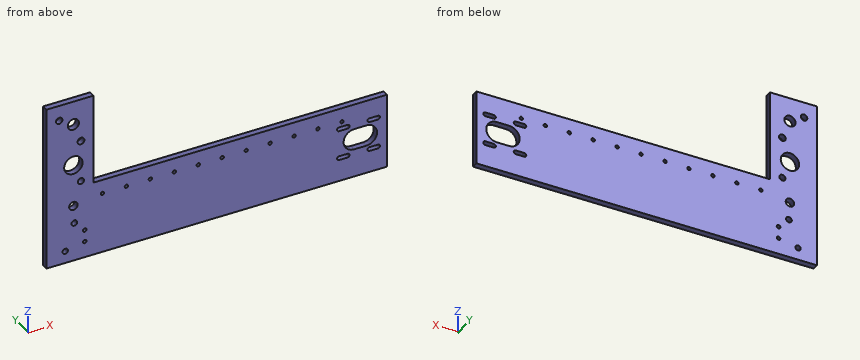
from build123d import *

# Parameters (mm, degrees)
BOSS_EXTRUDE1_DEPTH = 6.35
SKETCH2_R           = 2.979007601
CUT_EXTRUDE1_DEPTH  = 7.35
SKETCH3_R           = 4.400364859
SKETCH3_R_2         = 9.604356308
SKETCH3_R_3         = 5.866647912
SKETCH3_R_4         = 3.226485866
SKETCH3_R_5         = 3.595926688
SKETCH3_R_6         = 3.386947747
SKETCH3_R_7         = 2.817872048
SKETCH3_R_8         = 1.840203328
SKETCH3_R_9         = 1.930985623
CUT_EXTRUDE2_DEPTH  = 7.35
SKETCH4_R           = 1.778
CUT_EXTRUDE3_DEPTH  = 7.35


with BuildPart() as part:
    # Sketch1 → Boss-Extrude1 (new body)
    with BuildSketch(Plane(origin=(0, 0, 0), x_dir=(1, 0, 0), z_dir=(0, 1, 0))):
        Polygon((-177.8, -87.3125), (-177.8, 87.3125), (177.8, 87.3125), (177.8, 8.2677), (-128.5875, 8.2677), (-128.5875, -87.3125), align=None)
    extrude(amount=BOSS_EXTRUDE1_DEPTH)

    # Sketch2 → Cut-Extrude1 (cut, through all)
    with BuildSketch(Plane(origin=(0, 6.35, 0), x_dir=(1, 0, 0), z_dir=(0, 1, 0))):
        with BuildLine():
            Line((143.6116, 35.2552), (156.3116, 35.2552))
            ThreePointArc((156.3116, 35.2552), (167.4241, 46.3677), (156.3116, 57.4802))
            Line((156.3116, 57.4802), (143.6116, 57.4802))
            ThreePointArc((143.6116, 57.4802), (132.4991, 46.3677), (143.6116, 35.2552))
        make_face()
        with BuildLine():
            Line((159.4866, 60.1472), (168.376602437, 60.1472))
            ThreePointArc((168.376602437, 60.1472), (170.472102437, 62.2427), (168.376602437, 64.3382))
            Line((168.376602437, 64.3382), (159.486602437, 64.3382))
            ThreePointArc((159.486602437, 64.3382), (157.3911, 62.242701219), (159.4866, 60.1472))
        make_face()
        with BuildLine():
            ThreePointArc((159.486602437, 28.3972), (157.3911, 30.492698781), (159.4866, 32.5882))
            Line((159.4866, 32.5882), (168.376602437, 32.5882))
            ThreePointArc((168.376602437, 32.5882), (170.472102437, 30.4927), (168.376602437, 28.3972))
            Line((168.376602437, 28.3972), (159.486602437, 28.3972))
        make_face()
        with BuildLine():
            Line((127.7366, 60.1472), (136.626602437, 60.1472))
            ThreePointArc((136.626602437, 60.1472), (138.722102437, 62.2427), (136.626602437, 64.3382))
            Line((136.626602437, 64.3382), (127.736602437, 64.3382))
            ThreePointArc((127.736602437, 64.3382), (125.6411, 62.242701219), (127.7366, 60.1472))
        make_face()
        with BuildLine():
            Line((136.626602437, 28.3972), (127.736602437, 28.3972))
            ThreePointArc((127.736602437, 28.3972), (125.6411, 30.492698781), (127.7366, 32.5882))
            Line((127.7366, 32.5882), (136.626602437, 32.5882))
            ThreePointArc((136.626602437, 32.5882), (138.722102437, 30.4927), (136.626602437, 28.3972))
        make_face()
        with Locations((-148.4884, 46.3677)):
            Circle(SKETCH2_R)
    extrude(amount=-CUT_EXTRUDE1_DEPTH, mode=Mode.SUBTRACT)

    # Sketch3 → Cut-Extrude2 (cut, through all)
    with BuildSketch(Plane(origin=(0, 6.35, 0), x_dir=(1, 0, 0), z_dir=(0, 1, 0))):
        with Locations((-149.5425, 27.305)):
            Circle(SKETCH3_R)
        with Locations((-149.5425, -17.4625)):
            Circle(SKETCH3_R_2)
        with Locations((-149.5425, -62.23)):
            Circle(SKETCH3_R_3)
        with Locations((-141.63041575, 2.468910578)):
            Circle(SKETCH3_R_4)
        with Locations((-141.63041575, -41.536127476)):
            Circle(SKETCH3_R_5)
        with Locations((-164.313722824, -70.828896652)):
            Circle(SKETCH3_R_6)
        with Locations((-157.998667059, 74.512666328)):
            Circle(SKETCH3_R_7)
        with Locations((-137.701702146, 70.163316704)):
            Circle(SKETCH3_R_8)
        with Locations((-137.701702146, 57.549974441)):
            Circle(SKETCH3_R_9)
    extrude(amount=-CUT_EXTRUDE2_DEPTH, mode=Mode.SUBTRACT)

    # Sketch4 → Cut-Extrude3 (cut, through all)
    with BuildSketch(Plane(origin=(0, 6.35, 0), x_dir=(1, 0, 0), z_dir=(0, 1, 0))):
        with Locations((130.81, 23.1267)):
            Circle(SKETCH4_R)
        with Locations((105.81, 23.1267)):
            Circle(SKETCH4_R)
        with Locations((80.81, 23.1267)):
            Circle(SKETCH4_R)
        with Locations((55.81, 23.1267)):
            Circle(SKETCH4_R)
        with Locations((30.81, 23.1267)):
            Circle(SKETCH4_R)
        with Locations((5.81, 23.1267)):
            Circle(SKETCH4_R)
        with Locations((-19.19, 23.1267)):
            Circle(SKETCH4_R)
        with Locations((-44.19, 23.1267)):
            Circle(SKETCH4_R)
        with Locations((-69.19, 23.1267)):
            Circle(SKETCH4_R)
        with Locations((-94.19, 23.1267)):
            Circle(SKETCH4_R)
        with Locations((-119.19, 23.1267)):
            Circle(SKETCH4_R)
    extrude(amount=-CUT_EXTRUDE3_DEPTH, mode=Mode.SUBTRACT)


solid = part.part
Source: CAD feature listing. Evaluate the final solid. Frame: model axes, mm. Give positions to 0.01 mm unless a question says otherwise; leave off trailing zeros. Loops run counter-clockwise (first coordinate to the right, second up) from the corner with the lowest first, then second, coordinate; pieces in that order, holes last. Notation, with made-up numbers: (-37, 8.25) -> (-8, 8.25) arc R33 ccw to (-8, 42.25) -> close; hole circle Ø10 at (2.25, 71). An arc over 180 degrees is marked (long way). Use a Markdown table: item, result. Add a question column.
1) Section query A-A, the plane z = -39.5. Return the cut outline in (x, y).
2) First-contact query: pin 1 (3 mm diameter, centred on x = 30.81, z = -23.13, fed in from +Y). Flat tip, straight axial feed; report the tip coordinate or a pass-through.
3) Section query B-B, the plane x = 24. Return the cut outline in (y, z), then the cut area to 3 significant figures.
4) Section query C-C, the plane y = 3.75. Count the separate pieces of the cut face and the enclosed holes in it, then the cut area to 3 significant figures.
5) Line query: line 1 along Z through (x, y) = (-44.19, 3); line 2 along Z through (x, y) = (161, 5.75); line 3 along Z through (x, y) = (-150, 1.25). Output: solid intervals per line, ascending. Write a range as [from, to].
Numbers:
| question | item | result |
|---|---|---|
| 1 | outline | (-177.8, 0) -> (134.88, 0) -> (134.88, 6.35) -> (-177.8, 6.35) -> close; (165.05, 0) -> (177.8, 0) -> (177.8, 6.35) -> (165.05, 6.35) -> close |
| 2 | pin 1 | passes through |
| 3 | outline | (0, -87.31) -> (6.35, -87.31) -> (6.35, -8.27) -> (0, -8.27) -> close |
| 3 | area | 502 mm2 |
| 4 | separate pieces | 1 |
| 4 | enclosed holes | 26 |
| 4 | area | 31,200 mm2 |
| 5 | line 1 | z = [-87.31, -24.9], [-21.35, -8.27] |
| 5 | line 2 | z = [-87.31, -64.34], [-60.15, -56.44], [-36.29, -32.59], [-28.4, -8.27] |
| 5 | line 3 | z = [-87.31, -48.93], [-43.8, -31.68], [-22.93, 7.87], [27.06, 56.38], [68.08, 87.31] |
